Could you check a few things on this model? Use its own coordinates, in mm. Face numbers are marked on the shaded views. Coordinates: 2 decimals unless noted, no trailing zeros. Order: outer loops, then holes, each group sorted by start corner. A loop starts at its lowest first (then second) coordinate and runs counter-clockwise, first axis right, second up. Notation, with made-up numbers: M -2.75,73.5 L 35.25,73.5 A18 ccw 35.25,82.5 Z; hole C 5,32 d9. An arc over 180 degrees is marked long. Write item = value, one per line. Start each with the question number.
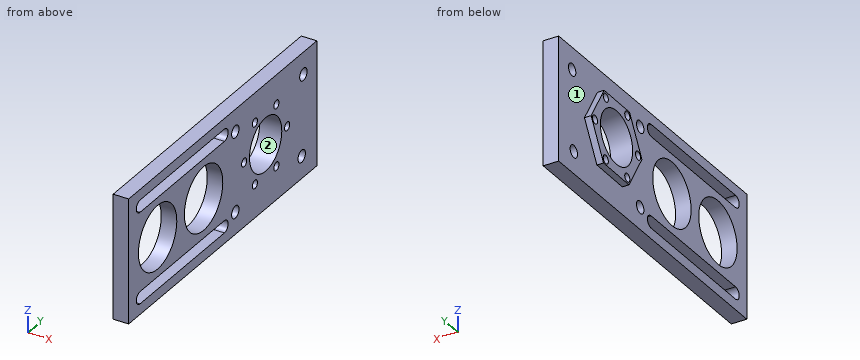
from build123d import *

# Parameters (mm, degrees)
SKETCH1_W           = 56
SKETCH1_H           = 140
BOSS_EXTRUDE1_DEPTH = 7
SKETCH2_R           = 14.275
SKETCH2_R_2         = 12
SKETCH2_R_3         = 1.9
CUT_EXTRUDE1_DEPTH  = 8
CUT_EXTRUDE2_DEPTH  = 8
SKETCH4_R           = 2.75
CUT_EXTRUDE3_DEPTH  = 8
BOSS_EXTRUDE3_DEPTH = 3
SKETCH8_R           = 1.9
SKETCH8_R_2         = 12
CUT_EXTRUDE5_DEPTH  = 4


with BuildPart() as part:
    # Sketch1 → Boss-Extrude1 (new body)
    with BuildSketch(Plane(origin=(0, 0, 0), x_dir=(0, 0, -1), z_dir=(1, 0, 0))):
        with Locations((28, 70)):
            Rectangle(SKETCH1_W, SKETCH1_H)
    extrude(amount=BOSS_EXTRUDE1_DEPTH)

    # Sketch2 → Cut-Extrude1 (cut, through all)
    with BuildSketch(Plane(origin=(7, 0, 0), x_dir=(0, 0, -1), z_dir=(1, 0, 0))):
        with Locations((28, 21.516289278)):
            Circle(SKETCH2_R)
        with Locations((28, 55.727598477)):
            Circle(SKETCH2_R)
        with Locations((27.137621846, 101.914121241)):
            Circle(SKETCH2_R_2)
        with Locations((40.994028307, 109.914121241)):
            Circle(SKETCH2_R_3)
        with Locations((27.137621846, 117.914121241)):
            Circle(SKETCH2_R_3)
        with Locations((13.281215386, 109.914121241)):
            Circle(SKETCH2_R_3)
        with Locations((40.994028307, 93.914121241)):
            Circle(SKETCH2_R_3)
        with Locations((27.137621846, 85.914121241)):
            Circle(SKETCH2_R_3)
        with Locations((13.281215386, 93.914121241)):
            Circle(SKETCH2_R_3)
    extrude(amount=-CUT_EXTRUDE1_DEPTH, mode=Mode.SUBTRACT)

    # Sketch3 → Cut-Extrude2 (cut, through all)
    with BuildSketch(Plane(origin=(7, 0, 0), x_dir=(0, 0, -1), z_dir=(1, 0, 0))):
        with BuildLine():
            Line((10.25, 71.244817418), (10.25, 8.434985259))
            ThreePointArc((10.25, 8.434985259), (7.5, 5.684985259), (4.75, 8.434985259))
            Line((4.75, 8.434985259), (4.75, 71.244817418))
            ThreePointArc((4.75, 71.244817418), (7.5, 73.994817418), (10.25, 71.244817418))
        make_face()
        with BuildLine():
            Line((45.75, 8.434985259), (45.75, 71.244817418))
            ThreePointArc((45.75, 71.244817418), (48.5, 73.994817418), (51.25, 71.244817418))
            Line((51.25, 71.244817418), (51.25, 8.434985259))
            ThreePointArc((51.25, 8.434985259), (48.5, 5.684985259), (45.75, 8.434985259))
        make_face()
    extrude(amount=-CUT_EXTRUDE2_DEPTH, mode=Mode.SUBTRACT)

    # Sketch4 → Cut-Extrude3 (cut, through all)
    with BuildSketch(Plane(origin=(7, 0, 0), x_dir=(0, 0, -1), z_dir=(1, 0, 0))):
        with Locations((10, 130)):
            Circle(SKETCH4_R)
        with Locations((46, 128.741828228)):
            Circle(SKETCH4_R)
        with Locations((46, 79.350819397)):
            Circle(SKETCH4_R)
        with Locations((10, 79.350819397)):
            Circle(SKETCH4_R)
    extrude(amount=-CUT_EXTRUDE3_DEPTH, mode=Mode.SUBTRACT)

    # Sketch7 → Boss-Extrude3 (add)
    with BuildSketch(Plane.ZY):
        Polygon((-10.64359884, 111.154642842), (-26.893136794, 120.818624975), (-43.3871598, 111.578103374), (-43.631644852, 92.673599639), (-27.382106898, 83.009617506), (-10.888083892, 92.250139107), align=None)
    extrude(amount=BOSS_EXTRUDE3_DEPTH)

    # Sketch8 → Cut-Extrude5 (cut, through all)
    with BuildSketch(Plane(origin=(0, 0, 0), x_dir=(0, 0, -1), z_dir=(1, 0, 0))):
        with Locations((13.281215386, 109.914121241)):
            Circle(SKETCH8_R)
        with Locations((13.281215386, 93.914121241)):
            Circle(SKETCH8_R)
        with Locations((27.137621846, 85.914121241)):
            Circle(SKETCH8_R)
        with Locations((40.994028307, 93.914121241)):
            Circle(SKETCH8_R)
        with Locations((40.994028307, 109.914121241)):
            Circle(SKETCH8_R)
        with Locations((27.137621846, 117.914121241)):
            Circle(SKETCH8_R)
        with Locations((27.137621846, 101.914121241)):
            Circle(SKETCH8_R_2)
    extrude(amount=-CUT_EXTRUDE5_DEPTH, mode=Mode.SUBTRACT)


solid = part.part
(1) Please list where these lines run through material, in increasing order: probe 1 along Z at (x, y) = (5, 93.5); probe 2 along Y at (x, z) = (1.25, -40); probe 3 along Y at (x, z) = (5.25, -15). Write a range as from..to.
(2) Imagine slicing it at D-D on z = -52.5. List the corners of the cut face in (x, y) for me.
(3) Imagine slicing it at A-A on y = 26. List the corners of the cut face in (x, z) for me, plus the area to 3 significant figures.
(4) Imagine slicing it at B-B on y = 130. List the corners of the cut face in (x, z) for me, plus the area to 3 significant figures.
(5) Thinking about a two-plate mould opening in Z: for the marked faces 1 and 2, which applies, released by +Z, released by -Z, zero draft, split by the parting line, or undercut?
(6) Imagine slicing it at C-C on x = 4.75. Give the number of separate pieces and of enclosed holes in the cut face, plus the area to 3 significant figures.
(7) Will these pins go through, and if not, where does the flat tip stop? P1, Ø3.5, axis at y = 93.91, z = -13.28, coming from the -X side; P2, Ø6.5, axis at y = 79.35, z = -46, coming from the -X side.
Response:
q1.probe_1 = -56..-42.85, -39.14..-35.69, -18.58..-15.14, -11.43..0
q1.probe_2 = 0..13.78, 29.25..48, 63.46..92.29, 95.53..108.29, 111.53..140
q1.probe_3 = 0..15.62, 27.41..49.83, 61.62..93.1, 94.72..109.1, 110.72..140
q2.outline = M 0,0 L 7,0 L 7,140 L 0,140 Z
q3.outline = M 0,-56 L 7,-56 L 7,-51.25 L 0,-51.25 Z; M 0,-45.75 L 7,-45.75 L 7,-41.55 L 0,-41.55 Z; M 0,-14.45 L 7,-14.45 L 7,-10.25 L 0,-10.25 Z; M 0,-4.75 L 7,-4.75 L 7,0 L 0,0 Z
q3.area = 125 mm2
q4.outline = M 0,-56 L 7,-56 L 7,-48.45 L 0,-48.45 Z; M 0,-43.55 L 7,-43.55 L 7,-12.75 L 0,-12.75 Z; M 0,-7.25 L 7,-7.25 L 7,0 L 0,0 Z
q4.area = 319 mm2
q5.face_1 = zero draft
q5.face_2 = undercut
q6.separate_pieces = 1
q6.enclosed_holes = 15
q6.area = 5,210 mm2
q7.P1 = through
q7.P2 = 0
